Part print with two shaded views. Sizes in mm from the minimum x, y, z corner. Round coordinates to 2 decimals unless told otherwise and drop trailing zeros. Loops run counter-clockwise (first coordinate to the right, second up) from the corner with the lowest first, then second, coordinate; pieces in that order, holes last. Notation, with made-up numbers: (3.5, 36.25) -> (32.5, 36.25) arc R30 ccw to (32.5, 61.25) -> close; hole circle Ø2 at (51, 41.25). An arc over 180 degrees is marked (long way). Answer as a JSON object with one key per item and string values. Group by question number.
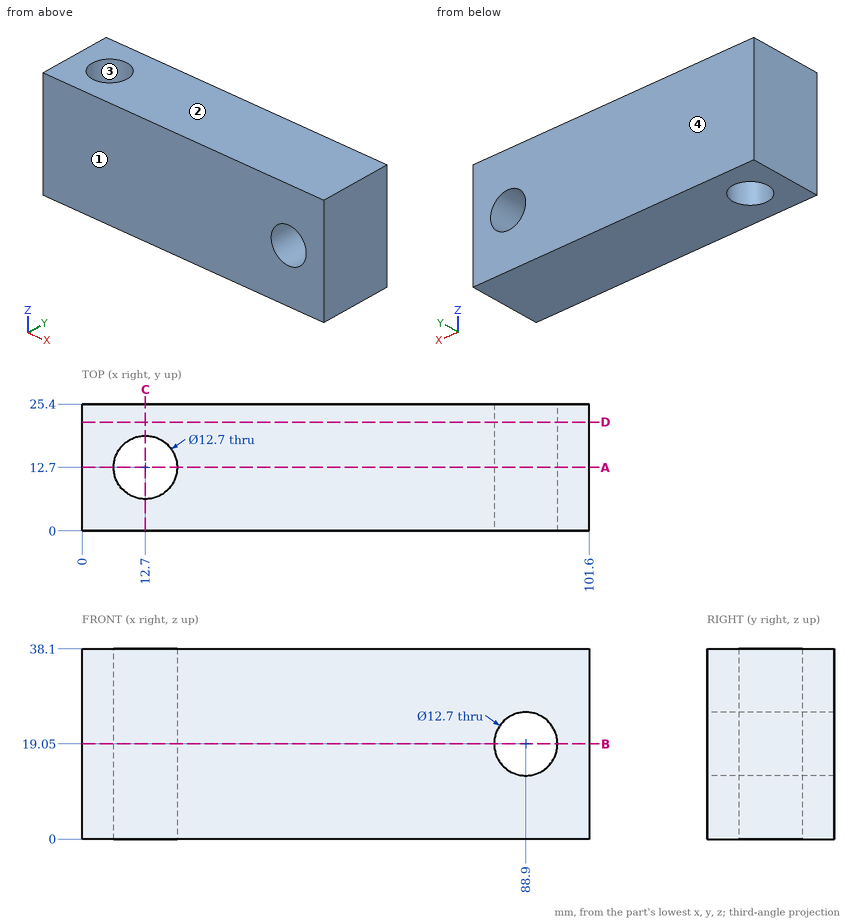
Item 1: Band-saw the part on A-A, the plane y = 12.7. List the corners of the cut face in (x, z).
Item 2: Drill centre lines: line 1 (Z direction, x = 88.9, y = 14.5); line 2 (Y direction, x = 12.7, z = 23); line 3 (Y direction, x = 8, z = 20.5). Where is each one in solid material? Low to high.
Item 3: Band-saw the part on D-D, the plane y = 21.75. List the corners of the cut face in (x, z).
Item 4: Two-plate mould, pull along Y, no slides. Class the marked faces 1, 2, 3 and 4: pulls with the +Y half, pulls with the -Y half, needs draft (parallel to the pull), parting line crosses it, or undercut.
Item 5: Band-saw the part on C-C, the plane x = 12.7. List the corners of the cut face in (y, z), plus the area to 3 significant figures.
Item 6: Band-saw the part on B-B, the plane z = 19.05. List the corners of the cut face in (x, y), plus the area to 3 significant figures.
Item 7: Drop a flat-ended pin along its axis: pin 1 Ø7.5 at (x, y) = (12.7, 12.7) entering from -Z. Give the stop position or say it passes through.
Entries:
{
 "1": {"outline": "(0, 0) -> (6.35, 0) -> (6.35, 38.1) -> (0, 38.1) -> close; (19.05, 0) -> (101.6, 0) -> (101.6, 38.1) -> (19.05, 38.1) -> close; hole circle Ø12.7 at (88.9, 19.05)"},
 "2": {"line 1": "0 to 12.7, 25.4 to 38.1", "line 2": "0 to 6.35, 19.05 to 25.4", "line 3": "0 to 8.43, 16.97 to 25.4"},
 "3": {"outline": "(0, 0) -> (101.6, 0) -> (101.6, 38.1) -> (0, 38.1) -> close; hole circle Ø12.7 at (88.9, 19.05)"},
 "4": {"face 1": "pulls with the -Y half", "face 2": "needs draft", "face 3": "undercut", "face 4": "pulls with the +Y half"},
 "5": {"outline": "(0, 0) -> (6.35, 0) -> (6.35, 38.1) -> (0, 38.1) -> close; (19.05, 0) -> (25.4, 0) -> (25.4, 38.1) -> (19.05, 38.1) -> close", "area": "484 mm²"},
 "6": {"outline": "(0, 0) -> (82.55, 0) -> (82.55, 25.4) -> (0, 25.4) -> close; (95.25, 0) -> (101.6, 0) -> (101.6, 25.4) -> (95.25, 25.4) -> close; hole circle Ø12.7 at (12.7, 12.7)", "area": "2,130 mm²"},
 "7": {"pin 1": "through"}
}
